Autodesk Inventor part; units mm, degrees
ref_plane "Work Plane2" through (0, 0, 2.5) normal (0, 0, 1) x (1, 0, 0)
ref_plane "Work Plane8" through (0, 0, 0) normal (0.9510565, 0.309017, 0) x (0, 0, 1)
ref_plane "Work Plane9" through (0, 0, 0) normal (1, 0, 0) x (0, 1, 0)
sketch "Sketch1" plane through (0, 0, 0) normal (0, 0, 1) x (1, 0, 0)
  circle A0 centre (0, 0) radius 3
  dimension "d0" = 6
extrude "Extrusion1" add sketch "Sketch1" along normal blind 5
ref_plane "Work Plane2" through (0, 0, 2.5) normal (0, 0, 1) x (1, 0, 0)
sketch "Sketch2" plane through (0, 0, 0) normal (0, 0, -1) x (-1, 0, 0)
  circle A0 centre (0, 0) radius 3
  circle A1 centre (0, 0) radius 2.5
  dimension "d3" = 5
surface extrude "Pitch Diameter" sketch "Sketch2" against normal through all shown no curves A1
ref_plane "Work Plane8" through (0, 0, 0) normal (0.9510565, 0.309017, 0) x (0, 0, 1)
ref_plane "Work Plane9" through (0, 0, 0) normal (1, 0, 0) x (0, 1, 0)
spur gear teeth "Spur Gear" teeth 10 pitch diameter 5 tip diameter 6 root diameter 3.75 face width 5 start plane through (0, 0, 0) normal (0, 0, -1) x (-1, 0, 0)
equation "\"d0\" = da_da"
equation "\"d1\" = da_b"
equation "\"d3\" = da_dw"
equation "\"d16\" = da_aw"
equation "\"d43\" = da_aw"
equation "\"d46\" = da_aw"
properties part number "Spur Gear1" material "Steel"
CAD build for the part. Positions are in the model's coordinates, mm. A direction names the side the tool comes from. Round coordinates to 2 decimals unless told otherwise and drop trailing zeros. Write each loop counter-clockwise with the first axis right and the second up, starting at its lowest first coordinate (ties: lowest second). Pieces come first, ordered by that corner, then holes. Notation, with made-up numbers: M 6,40 L 17,40 A33 ccw 17,71 Z; hole C 4.25,88 d7. An arc over 180 degrees is marked long. Use a Markdown table: item, result. Add a question column.
1. Slice it at A-A on x = 2.6. Give the cut face in (y, z), then the cut area to 3 significant figures.
2. Drill centre lines: probe 1 along Y at (x, z) = (1.8, 4.4); probe 2 along X at (y, z) = (-1.9, 1.7); probe 3 along X at (y, z) = (-2.5, 4.8). Where is each one in solid material? Low to high.
3. Slice it at B-B on x = -1.7. Give the cut face in (y, z).
4. Flat gauge pin, fed straight in: P1, Ø1, axis at y = 0, z = 1.5, coming from the +X side. Where does the tip first touch, or does it go through?
5. Slice it at D-D on x = 0.8. Give the cut face in (y, z).
6. 3-axis set-ups, long thin cutter, end or side, ignore diameter. For faces 4 (the face through (2.18, -1.13, 2.46)), 5 (the face through (2.43, 0.37, 2.46)), 6 (the face through (1.103, -2.197, 2.465)), 7 (the face through (0, 0, 5)), 8 (the face through (-1.74, 1.71, 2.46)): which of +Z, -Z, +X, -X, +Y, -Y reach the whole face in a straight line?
7. Pull direction Y, two halves, no side cores. Call faces 1 (the face through (1.091, 2.186, 2.465)), 2 (the face through (-1.091, -2.186, 2.465)), 3 (the face through (-2.416, 0.362, 2.465)): released by +Y, released by -Y, zero draft, split by the parting line, or undercut.
8. Slice it at C-C on y = -1.3. Give the cut face in (x, z), then the cut area to 3 significant figures.
Reply:
| question | item | result |
|---|---|---|
| 1 | outline | M -1.16,0 L -0.47,0 L -0.47,5 L -1.16,5 Z; M 0.47,0 L 1.16,0 L 1.16,5 L 0.47,5 Z |
| 1 | area | 6.87 mm^2 |
| 2 | probe 1 | y = -2.4 to -1.84, -1.05 to 1.05, 1.84 to 2.4 |
| 2 | probe 2 | x = -1.83 to -0.84, -0.44 to 0.44, 0.84 to 1.83 |
| 2 | probe 3 | x = -1.66 to -1.48, -0.38 to 0.38, 1.48 to 1.66 |
| 3 | outline | M -2.47,0 L -1.63,0 L -1.63,5 L -2.47,5 Z; M -1.02,0 L 1.02,0 L 1.02,5 L -1.02,5 Z; M 1.63,0 L 2.47,0 L 2.47,5 L 1.63,5 Z |
| 4 | P1 | stops at x = 2.65 |
| 5 | outline | M -1.85,0 L 1.85,0 L 1.85,5 L -1.85,5 Z |
| 6 | face 4 | +Z, -Z |
| 6 | face 5 | +Z, -Z, +X |
| 6 | face 6 | +Z, -Z, -Y |
| 6 | face 7 | +Z, +X, -X, +Y, -Y |
| 6 | face 8 | +Z, -Z, -X |
| 7 | face 1 | released by +Y |
| 7 | face 2 | released by -Y |
| 7 | face 3 | undercut |
| 8 | outline | M -1.49,0 L 1.49,0 L 1.49,5 L -1.49,5 Z |
| 8 | area | 14.9 mm^2 |
